Design review of the part built by this model. Coordinates are the model's own, in mm. Face numbers are marked on the shaded views. A direction names the side the tool comes from. Give positions to 0.01 mm unless a question says otherwise; leave off trailing zeros. Loops run counter-clockwise (first coordinate to the right, second up) from the corner with the lowest first, then second, coordinate; pieces in that order, holes last. Notation, with made-up numbers: (43, 2.25) -> (74, 2.25) arc R17 cw to (74, 27.25) -> close; hole circle Ø4 at (49, 38). An arc over 180 degrees is marked (long way). Use a Markdown table: item, result. Add a question column.
1. For pin 1 Ø8 at (x, y) = (23, 10.5) entering from +Z; pin 2 Ø2 at (x, y) = (11.5, 17) entering from -Z; pin 3 Ø1.5 at (x, z) = (29, -5) entering from +Y, all flat-tipped, find the tip position at first contact; note any pin that passes through.
2. Add section A-A (x = 27). State the section outline as (y, z) points.
3. Add section D-D (z = 6.25). State the section outline as (x, y) points, and give its area (3 significant figures).
4. To check wall thickness, follow line 1 (Y direction, x = 24.5, z = 1.8); line 2 (Y direction, x = 2, z = 1.75); line 3 (Y direction, x = 7.5, z = -7.75). State the ranges of each line that lie inside material, in increasing order.
5. Add section C-C (y = 24.5). State the section outline as (x, z) points.
6. For the marked faces 4, 5 and 6, list the 3-axis set-ups (+Z, -Z, +X, -X, +Y, -Y) from which the entire face can be reached by the end or side of a thin tool; tool diameter is ignored.
7. Draft analysis for pull direction X (two halves, no side actions). For the marked faces 1, 2 and 3, state which applies: pulls with the +X half, pulls with the -X half, needs draft (parallel to the pull), parting line crosses it, or undercut.
8. Add section B-B (z = -4). State the section outline as (x, y) points.
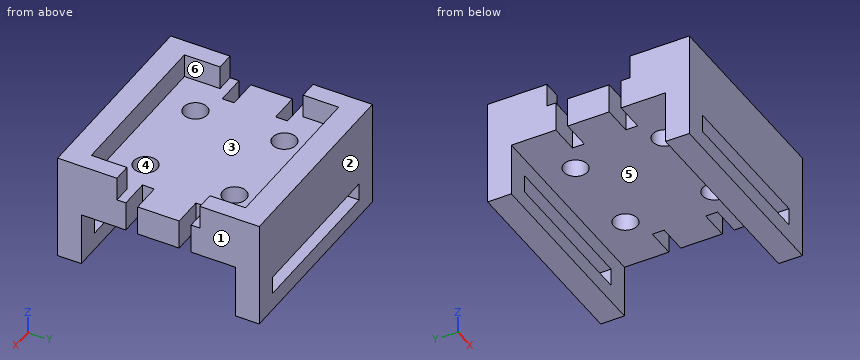
```python
from build123d import *

# Parameters (mm, degrees)
SKETCH1_W          = 34
SKETCH1_H          = 34
SKETCH1_R          = 2
BODY_DEPTH         = 5
SKETCH2_W          = 34
SKETCH2_H          = 4
LEG1_DEPTH         = 3
SKETCH3_W          = 4
SKETCH3_H          = 4
LEG2_DEPTH         = 3
SKETCH4_W          = 34
SKETCH4_H          = 4
LEG3_DEPTH         = 3
WALLS_DEPTH        = 4
SKETCH6_W          = 5
SKETCH6_H          = 2
CUT_EXTRUDE1_DEPTH = 5


with BuildPart() as part:
    # Sketch1 → Body (new body)
    with BuildSketch(Plane.XY):
        with Locations((17, 17)):
            Rectangle(SKETCH1_W, SKETCH1_H)
        with Locations((24.5, 24.5)):
            Circle(SKETCH1_R, mode=Mode.SUBTRACT)
        with Locations((9.5, 24.5)):
            Circle(SKETCH1_R, mode=Mode.SUBTRACT)
        with Locations((9.5, 9.5)):
            Circle(SKETCH1_R, mode=Mode.SUBTRACT)
        with Locations((24.5, 9.5)):
            Circle(SKETCH1_R, mode=Mode.SUBTRACT)
    extrude(amount=BODY_DEPTH)

    # Sketch2 → Leg1 (add)
    with BuildSketch(Plane(origin=(0, 0, 0), x_dir=(-1, 0, 0), z_dir=(0, 0, -1))):
        with Locations((-17, 32)):
            Rectangle(SKETCH2_W, SKETCH2_H)
        with Locations((-17, 2)):
            Rectangle(SKETCH2_W, SKETCH2_H)
    extrude(amount=LEG1_DEPTH)

    # Sketch3 → Leg2 (add)
    with BuildSketch(Plane(origin=(0, 0, -3), x_dir=(-1, 0, 0), z_dir=(0, 0, -1))):
        with Locations((-32, 32)):
            Rectangle(SKETCH3_W, SKETCH3_H)
        with Locations((-2, 32)):
            Rectangle(SKETCH3_W, SKETCH3_H)
        with Locations((-2, 2)):
            Rectangle(SKETCH3_W, SKETCH3_H)
        with Locations((-32, 2)):
            Rectangle(SKETCH3_W, SKETCH3_H)
    extrude(amount=LEG2_DEPTH)

    # Sketch4 → Leg3 (add)
    with BuildSketch(Plane(origin=(0, 0, -6), x_dir=(-1, 0, 0), z_dir=(0, 0, -1))):
        with Locations((-17, 32)):
            Rectangle(SKETCH4_W, SKETCH4_H)
        with Locations((-17, 2)):
            Rectangle(SKETCH4_W, SKETCH4_H)
    extrude(amount=LEG3_DEPTH)

    # Sketch5 → Walls (add)
    with BuildSketch(Plane.XY.offset(5)):
        Polygon((0, 34), (34, 34), (34, 30), (34, 24), (31, 24), (31, 30), (3, 30), (3, 24), (0, 24), (0, 30), align=None)
        Polygon((31, 10), (34, 10), (34, 4), (34, 0), (0, 0), (0, 4), (0, 10), (3, 10), (3, 4), (31, 4), align=None)
    extrude(amount=WALLS_DEPTH)

    # Sketch6 → Cut-Extrude1 (cut)
    with BuildSketch(Plane.XY.offset(5)):
        with Locations((2.5, 21.5)):
            Rectangle(SKETCH6_W, SKETCH6_H)
        with Locations((31.5, 21.5)):
            Rectangle(SKETCH6_W, SKETCH6_H)
        with Locations((2.5, 12.5)):
            Rectangle(SKETCH6_W, SKETCH6_H)
        with Locations((31.5, 12.5)):
            Rectangle(SKETCH6_W, SKETCH6_H)
    extrude(amount=-CUT_EXTRUDE1_DEPTH, mode=Mode.SUBTRACT)


solid = part.part
```
Taken from the geometry:
| question | item | result |
|---|---|---|
| 1 | pin 1 | stops at z = 5 |
| 1 | pin 2 | stops at z = 0 |
| 1 | pin 3 | passes through |
| 2 | outline | (0, -9) -> (4, -9) -> (4, -6) -> (0, -6) -> close; (0, -3) -> (4, -3) -> (4, 0) -> (30, 0) -> (30, -3) -> (34, -3) -> (34, 9) -> (30, 9) -> (30, 5) -> (4, 5) -> (4, 9) -> (0, 9) -> close; (30, -9) -> (34, -9) -> (34, -6) -> (30, -6) -> close |
| 3 | outline | (0, 0) -> (34, 0) -> (34, 10) -> (31, 10) -> (31, 4) -> (3, 4) -> (3, 10) -> (0, 10) -> close; (0, 24) -> (3, 24) -> (3, 30) -> (31, 30) -> (31, 24) -> (34, 24) -> (34, 34) -> (0, 34) -> close |
| 3 | area | 344 mm^2 |
| 4 | line 1 | y = 0 to 7.5, 11.5 to 22.5, 26.5 to 34 |
| 4 | line 2 | y = 0 to 11.5, 13.5 to 20.5, 22.5 to 34 |
| 4 | line 3 | y = 0 to 4, 30 to 34 |
| 5 | outline | (0, 0) -> (7.5, 0) -> (7.5, 5) -> (3, 5) -> (3, 9) -> (0, 9) -> close; (11.5, 0) -> (22.5, 0) -> (22.5, 5) -> (11.5, 5) -> close; (26.5, 0) -> (34, 0) -> (34, 9) -> (31, 9) -> (31, 5) -> (26.5, 5) -> close |
| 6 | face 4 | +Z, -Z |
| 6 | face 5 | -Z, +X, -X |
| 6 | face 6 | +Z |
| 7 | face 1 | pulls with the +X half |
| 7 | face 2 | needs draft |
| 7 | face 3 | undercut |
| 8 | outline | (0, 0) -> (4, 0) -> (4, 4) -> (0, 4) -> close; (0, 30) -> (4, 30) -> (4, 34) -> (0, 34) -> close; (30, 0) -> (34, 0) -> (34, 4) -> (30, 4) -> close; (30, 30) -> (34, 30) -> (34, 34) -> (30, 34) -> close |
